```python
from build123d import *

# Parameters (mm, degrees)
SKETCH1_R           = 2.4
SKETCH1_R_2         = 2.5
BOSS_EXTRUDE1_DEPTH = 3


with BuildPart() as part:
    # Sketch1 → Boss-Extrude1 (new body)
    # profile 1 of 4: a face of its own
    with BuildSketch(Plane(origin=(0, 0, 0), x_dir=(1, 0, 0), z_dir=(0, 1, 0))):
        with BuildLine():
            Line((19.068769591, 26.574235382), (19.068769591, -48.425764618))
            ThreePointArc((19.068769591, -48.425764618), (24.068769591, -53.425764618), (29.068769591, -48.425764618))
            Line((29.068769591, -48.425764618), (29.068769591, 21.574235382))
            Line((29.068769591, 21.574235382), (24.068769591, 21.574235382))
            Line((24.068769591, 21.574235382), (24.068769591, 24.074235382))
            ThreePointArc((24.068769591, 24.074235382), (22.301002638, 24.806468429), (21.568769591, 26.574235382))
            Line((21.568769591, 26.574235382), (19.068769591, 26.574235382))
        make_face()
        with Locations(Location((24.068769591, -48.425764618, 0), (0, 0, 270))):
            Circle(SKETCH1_R, mode=Mode.SUBTRACT)
    # profile 2 of 4: a face of its own
    with BuildSketch(Plane(origin=(0, 0, 0), x_dir=(1, 0, 0), z_dir=(0, 1, 0))):
        with BuildLine():
            Line((44.068769591, 31.574235382), (24.068769591, 31.574235382))
            Line((24.068769591, 31.574235382), (24.068769591, 29.074235382))
            ThreePointArc((24.068769591, 29.074235382), (25.836536544, 28.342002335), (26.568769591, 26.574235382))
            Line((26.568769591, 26.574235382), (29.068769591, 26.574235382))
            Line((29.068769591, 26.574235382), (29.068769591, 21.574235382))
            Line((29.068769591, 21.574235382), (44.068769591, 21.574235382))
            ThreePointArc((44.068769591, 21.574235382), (49.068769591, 26.574235382), (44.068769591, 31.574235382))
        make_face()
        with Locations(Location((44.068769591, 26.574235382, 0), (0, 0, 270))):
            Circle(SKETCH1_R_2, mode=Mode.SUBTRACT)
    # profile 3 of 4: a face of its own
    with BuildSketch(Plane(origin=(0, 0, 0), x_dir=(1, 0, 0), z_dir=(0, 1, 0))):
        with BuildLine():
            Line((24.068769591, 21.574235382), (29.068769591, 21.574235382))
            Line((29.068769591, 21.574235382), (29.068769591, 26.574235382))
            Line((29.068769591, 26.574235382), (26.568769591, 26.574235382))
            ThreePointArc((26.568769591, 26.574235382), (25.836536544, 24.806468429), (24.068769591, 24.074235382))
            Line((24.068769591, 24.074235382), (24.068769591, 21.574235382))
        make_face()
    # profile 4 of 4: a face of its own
    with BuildSketch(Plane(origin=(0, 0, 0), x_dir=(1, 0, 0), z_dir=(0, 1, 0))):
        with BuildLine():
            ThreePointArc((24.068769591, 31.574235382), (20.533235685, 30.109769288), (19.068769591, 26.574235382))
            Line((19.068769591, 26.574235382), (21.568769591, 26.574235382))
            ThreePointArc((21.568769591, 26.574235382), (22.301002638, 28.342002335), (24.068769591, 29.074235382))
            Line((24.068769591, 29.074235382), (24.068769591, 31.574235382))
        make_face()
    extrude(amount=BOSS_EXTRUDE1_DEPTH)


solid = part.part
```
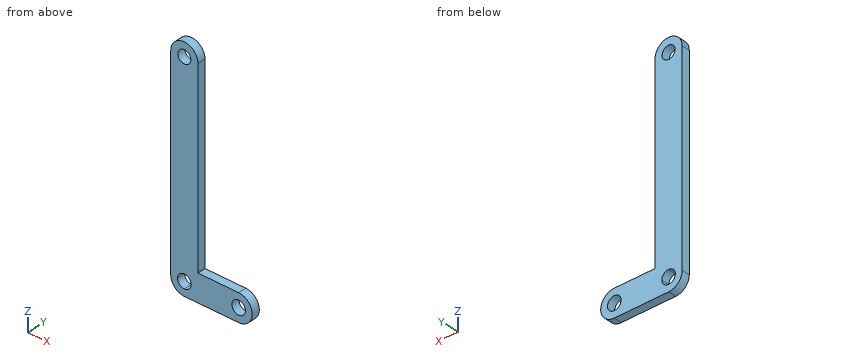
Here's how the part is built. I have some questions about the finished solid (model axes, mm). Give positions to 0.01 mm unless a question says otherwise; leave off trailing zeros. Loops run counter-clockwise (first coordinate to the right, second up) from the corner with the lowest first, then second, coordinate; pieces in that order, holes last. Notation, with made-up numbers: (62.25, -17) -> (98.25, -17) arc R36 ccw to (98.25, 17) -> close; hole circle Ø11 at (6.5, -13.75). An arc over 180 degrees is marked (long way). Use one line per item in the form item = value. Start each with the question number.
1) Imagine slicing it at B-B (x = 42.5). Please give me the cut outline in (y, z).
2) Imagine slicing it at D-D (x = 33.25). Please give me the cut outline in (y, z), then the cut area to 3 significant figures.
3) Imagine slicing it at A-A (y = 2.55). Please give me the cut outline in (x, z).
4) Imagine slicing it at C-C (z = 41). Please give me the cut outline in (x, y), then the cut area to 3 significant figures.
5) For P1, Ø0.9, axis at y = 1.5, z = -2.5, coming from the +X side; P2, Ø8, axis at x = 44.07, z = -26.57, coming from the +Y side; P3, Ø1.5, axis at x = 35.5, y = 2, coming from the +Z side, each with a flat end and sliding along its axis, tell me the tip position at first contact or that it passes through.
6) Please list where these lines run through material, in increasing order: line 1 along Z through (x, y) = (24.5, 2.4); line 2 along X through (y, z) = (1.85, -11); line 3 along Z through (x, y) = (24.75, 0.3).
Check values:
q1.outline = (0, -31.57) -> (3, -31.57) -> (3, -28.52) -> (0, -28.52) -> close; (0, -24.63) -> (3, -24.63) -> (3, -21.57) -> (0, -21.57) -> close
q2.outline = (0, -31.57) -> (3, -31.57) -> (3, -21.57) -> (0, -21.57) -> close
q2.area = 30.0 mm^2
q3.outline = (19.07, -26.57) arc R5 ccw to (24.07, -31.57) -> (44.07, -31.57) arc R5 ccw to (44.07, -21.57) -> (29.07, -21.57) -> (29.07, 48.43) arc R5 ccw to (19.07, 48.43) -> close; hole circle Ø5 at (24.07, -26.57); hole circle Ø4.8 at (24.07, 48.43); hole circle Ø5 at (44.07, -26.57)
q4.outline = (19.07, 0) -> (29.07, 0) -> (29.07, 3) -> (19.07, 3) -> close
q4.area = 30.0 mm^2
q5.P1 = 29.07
q5.P2 = 3
q5.P3 = -21.57
q6.line_1 = -31.57 to -29.04, -24.11 to 46.06, 50.79 to 53.41
q6.line_2 = 19.07 to 29.07
q6.line_3 = -31.57 to -28.98, -24.17 to 46.12, 50.73 to 53.38
